```python
from build123d import *

# Parameters (mm, degrees)
F0_W      = 40
F0_H      = 155
F0_W_2    = 10
F0_H_2    = 37
F1_DEPTH  = 5
F2_R      = 4.99999
F3_W      = 20
F3_H      = 47
F4_DEPTH  = 20
F5_R      = 5
F6_SIZE   = 4.99999
F7_R      = 2.074
F8_DEPTH  = 25.001
F9_W      = 5
F9_H      = 30
F10_DEPTH = 25.001
F11_R     = 2.49999


# Not quite as in the source:
# - a fillet or chamfer is up to 0.001 mm smaller than in the source, because OpenCascade refuses the exact size
# - ends of sketch curves that miss each other by under 0.0002 mm in the source are joined


with BuildPart() as f1:
    # F0 (on Top) → F1 (new body)
    with BuildSketch(Plane.XY):
        with Locations((0, 20)):
            Rectangle(F0_W, F0_H)
        with Locations((0, 54)):
            Rectangle(F0_W_2, F0_H_2, mode=Mode.SUBTRACT)
    extrude(amount=F1_DEPTH)

    # F2 (radius 5 in the source; OpenCascade refuses exactly that, so slightly less here)
    f2_edges = [f1.edges().sort_by_distance(p)[0] for p in [
        (5, 72.5, 2.5),
        (-5, 72.5, 2.5),
        (5, 35.5, 2.5),
        (-5, 35.5, 2.5),
    ]]
    fillet(f2_edges, radius=F2_R)

    # F3 (on face) → F4 (join)
    with BuildSketch(Plane(origin=(0, 0, 0), x_dir=(1, 0, 0), z_dir=(0, 0, -1))):
        with Locations((0, -54)):
            Rectangle(F3_W, F3_H)
        with BuildLine():
            ThreePointArc((-1e-05, -72.5), (-3.5355368349, -71.0355368349), (-5, -67.50001))
            Line((-5, -67.50001), (-5, -40.49999))
            ThreePointArc((-5, -40.49999), (-3.5355368349, -36.9644631651), (-1e-05, -35.5))
            ThreePointArc((-1e-05, -35.5), (3.5355368349, -36.9644631651), (5, -40.49999))
            Line((5, -40.49999), (5, -67.50001))
            ThreePointArc((5, -67.50001), (3.5355368349, -71.0355368349), (-1e-05, -72.5))
        make_face(mode=Mode.SUBTRACT)
    extrude(amount=F4_DEPTH)

    # F5
    f5_edges = [f1.edges().sort_by_distance(p)[0] for p in [
        (-10, 30.5, -10),
        (10, 30.5, -10),
        (-10, 77.5, -10),
        (10, 77.5, -10),
    ]]
    fillet(f5_edges, radius=F5_R)

    # F6 (size 5 in the source; OpenCascade refuses exactly that, so slightly less here)
    f6_edges = [f1.edges().sort_by_distance(p)[0] for p in [
        (0, 97.5, 0),
        (0, -57.5, 0),
    ]]
    chamfer(f6_edges, length=F6_SIZE)

    # F7 (on face) → F8 (cut, through all)
    with BuildSketch(Plane.XY.offset(5)):
        with Locations((-12.5, -42.5)):
            Circle(F7_R)
        with Locations((12.5, -42.5)):
            Circle(F7_R)
        with Locations((-12.5, -22.5)):
            Circle(F7_R)
        with Locations((12.5, -22.5)):
            Circle(F7_R)
        with Locations((-12.5, -2.5)):
            Circle(F7_R)
        with Locations((12.5, -2.5)):
            Circle(F7_R)
        with Locations((-12.5, 17.5)):
            Circle(F7_R)
        with Locations((12.5, 17.5)):
            Circle(F7_R)
        with Locations((-12.5, 37.5)):
            Circle(F7_R)
        with Locations((12.5, 37.5)):
            Circle(F7_R)
        with Locations((12.5, 57.5)):
            Circle(F7_R)
        with Locations((-12.5, 57.5)):
            Circle(F7_R)
        with Locations((12.5, 77.5)):
            Circle(F7_R)
        with Locations((-12.5, 77.5)):
            Circle(F7_R)
    extrude(amount=-F8_DEPTH, mode=Mode.SUBTRACT)

    # F9 (on face) → F10 (cut, through all)
    with BuildSketch(Plane.XY.offset(5)):
        with Locations((0, -31.5)):
            Rectangle(F9_W, F9_H)
    extrude(amount=-F10_DEPTH, mode=Mode.SUBTRACT)

    # F11 (radius 2.5 in the source; OpenCascade refuses exactly that, so slightly less here)
    f11_edges = [f1.edges().sort_by_distance(p)[0] for p in [
        (-2.5, -46.5, 2.5),
        (2.5, -46.5, 2.5),
        (-2.5, -16.5, 2.5),
        (2.5, -16.5, 2.5),
    ]]
    fillet(f11_edges, radius=F11_R)


solid = f1.part
```
Model file for the job. Use its own axes, mm. A direction names the side the tool comes from. Give positions to 0.01 mm unless a question says otherwise; leave off trailing zeros. Loops run counter-clockwise (first coordinate to the right, second up) from the corner with the lowest first, then second, coordinate; pieces in that order, holes last. Notation, with made-up numbers: (11.5, -20) -> (60.5, -20) arc R26 ccw to (60.5, 8) -> close; hole circle Ø7 at (18.5, -6). An arc over 180 degrees is marked (long way). Use CSV: the item, a comma, the result in double quotes. Start each with the question number.
1) Tool access for faces 4 (the flat face through (-7, 54, -20)), 5 (the cylindrical face through (-1.748, -17.213, 2.465)), 6 (the flat face through (-10, 54, -10)), 7 (the cylindrical face through (8.5, 31.93, -10.14)), 8 (the flat face through (10, 54, -10)): list every direction of +Z, -Z, +X, -X, +Y, -Y with a clear straight run to the whole face (end or side of a thin tool).
2) Slice it at B-B on z = -3.25. Give the cut face in (x, y), plus the area to 3 significant figures.
3) Slice it at A-A on x = -12.5. Give the number of separate pieces and of enclosed holes in the cut face, plus the area to 3 significant figures.
4) Wall check: line 1 (Y direction, x = 0, z = -16.75); line 2 (X direction, y = -36, z = 3.75); line 3 (X direction, y = 56.5, z = -3). Give the ranges that are in metal, low to high.
5) Mould opens along X. For faces 1 (the cylindrical face through (-8.57, 32, -10.14)), 2 (the flat face through (0, 21, 5)), 3 (the cylindrical face through (-11.54, 55.66, 2.54)) say: released by +X, released by -X, zero draft, split by the parting line, or undercut.
6) Slice it at D-D on y = 63. Give the cut face in (x, z), plus the area to 3 significant figures.
7) Flat gauge pins, fed straight in: pin 1 Ø1.5 at (x, z) = (2, -5) entering from +Y; pin 2 Ø5 at (x, z) = (0, -7.5) entering from -Y; pin 3 Ø12.5 at (y, z) = (53.5, -13.5) entering from +X; pin 4 Ø3.5 at (x, y) = (-12.5, 37.5) entering from +Z. Where does each tip first touch, or does it go through?
8) Slice it at C-C on y = 17.5. Give the cut face in (x, z).
Computed values:
1,face 4,"-Z, +X, -X, +Y, -Y"
1,face 5,"+Z, -Z"
1,face 6,"-Z, -X, +Y, -Y"
1,face 7,"-Z, +X, -Y"
1,face 8,"-Z, +X, +Y, -Y"
2,outline,"(-10, 35.5) arc R5 ccw to (-5, 30.5) -> (5, 30.5) arc R5 ccw to (10, 35.5) -> (10, 72.5) arc R5 ccw to (5, 77.5) -> (-5, 77.5) arc R5 ccw to (-10, 72.5) -> close; hole (-5, 40.5) arc R5 ccw to (0, 35.5) arc R5 ccw to (5, 40.5) -> (5, 67.5) arc R5 ccw to (0, 72.5) arc R5 ccw to (-5, 67.5) -> close"
2,area,"570 mm^2"
3,separate pieces,"8"
3,enclosed holes,"0"
3,area,"605 mm^2"
4,line 1,"y = 30.5 to 35.5, 72.5 to 77.5"
4,line 2,"x = -20 to -2.5, 2.5 to 20"
4,line 3,"x = -10 to -5, 5 to 10"
5,face 1,"released by -X"
5,face 2,"zero draft"
5,face 3,"undercut"
6,outline,"(-20, 0) -> (-10, 0) -> (-10, -20) -> (-5, -20) -> (-5, 5) -> (-20, 5) -> close; (5, -20) -> (10, -20) -> (10, 0) -> (20, 0) -> (20, 5) -> (5, 5) -> close"
6,area,"350 mm^2"
7,pin 1,"stops at y = 77.5"
7,pin 2,"stops at y = 30.5"
7,pin 3,"stops at x = 10"
7,pin 4,"passes through"
8,outline,"(-20, 0) -> (-14.57, 0) -> (-14.57, 5) -> (-20, 5) -> close; (-10.43, 0) -> (10.43, 0) -> (10.43, 5) -> (-10.43, 5) -> close; (14.57, 0) -> (20, 0) -> (20, 5) -> (14.57, 5) -> close"
